Can you work these out from the drawing? Everything is in mm from the part's minimum corner. Round coordinates to 2 decimals unless told otherwise and drop trailing zeros. Write each loop counter-clockwise with the first axis right and the second up, starting at its lowest first coordinate (ties: lowest second). Pieces come first, ordered by that corner, then holes. Notation, with made-up numbers: (-1, 19.25) -> (49, 19.25) arc R18 cw to (49, 36.25) -> close; hole circle Ø9 at (47.25, 6.25). An arc over 180 degrees is marked (long way). Put each result on its own line as item: value. Start each with the question number.
1. For pin 1 (8 mm diameter, centred on x = 230, y = 12, fed in from -Z); pin 2 (6 mm diameter, centred on y = 7.5, z = 337, fed in from +X); pin 3 (5 mm diameter, centred on y = 18, z = 234.5, fed in from +X); pin 4 (12 mm diameter, centred on x = 177.5, z = 104, fed in from +Y), each with a flat end and sliding along its axis, tell me the tip position at first contact or that it passes through.
2. I need wall thicknesses on probe 1 along Z at (x, y) = (294.5, 10.5); probe 2 along X at (y, z) = (12.5, 242.5); probe 3 along Z at (x, y) = (364, 19.5). Which ranges of each line are inside material? Lowest first, please. Write a range as from..to.
3. Suppose I cut it at C-C (y = 17). Please give me the cut outline in (x, z), then the cut area to 3 significant figures.
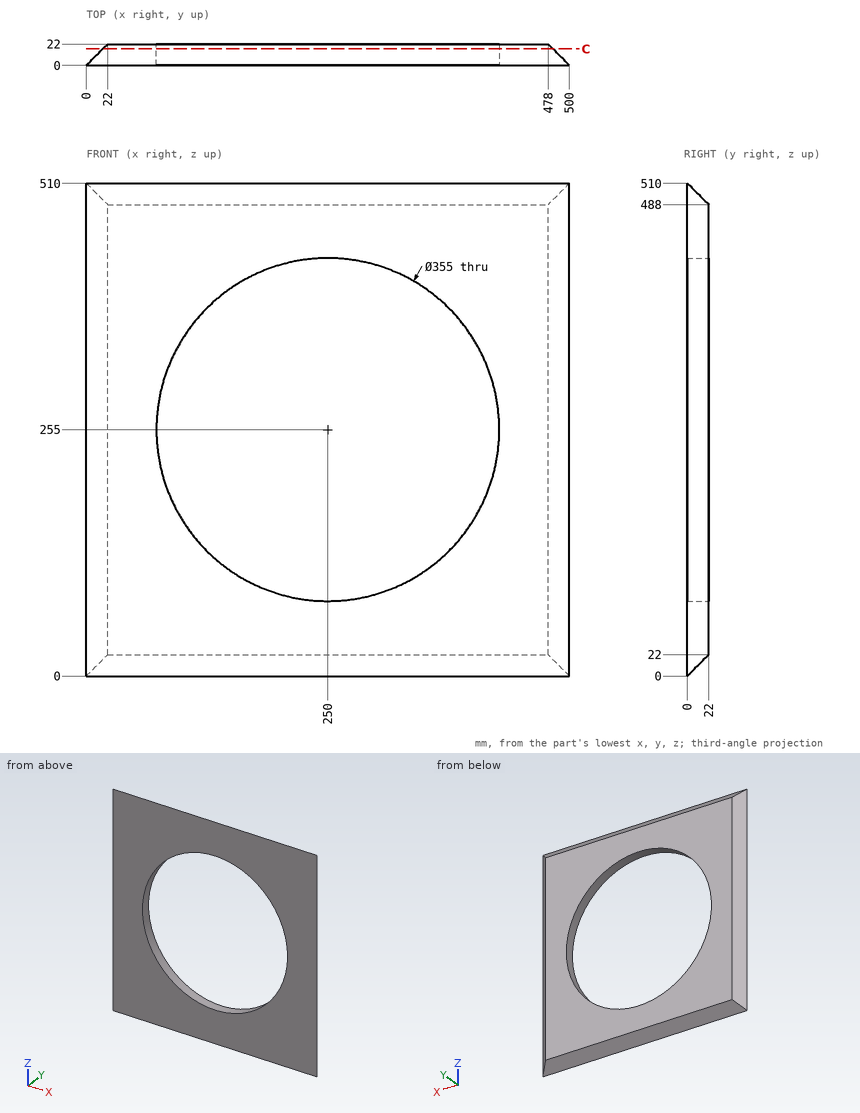
Verdict:
1. pin 1: stops at z = 8
1. pin 2: stops at x = 495.5
1. pin 3: stops at x = 484.5
1. pin 4: passes through
2. probe 1: z = 10.5..83.17, 426.83..499.5
2. probe 2: x = 12.5..72.94, 427.06..487.5
2. probe 3: z = 19.5..118.95, 391.05..490.5
3. outline: (17, 17) -> (483, 17) -> (483, 493) -> (17, 493) -> close; hole circle Ø355 at (250, 255)
3. area: 123,000 mm^2
